from build123d import *

# Parameters (mm, degrees)
EXTRUDE_1_DEPTH     = 20
SKETCH_2_R          = 3.25
CUT_EXTRUDE_1_DEPTH = 115.891252931
SKETCH_3_R          = 3.25
CUT_EXTRUDE_2_DEPTH = 115.891252931
CUT_EXTRUDE_3_DEPTH = 115.891252931
SKETCH_7_R          = 5.5
CUT_EXTRUDE_4_DEPTH = 25
SKETCH_8_R          = 5.5
CUT_EXTRUDE_5_DEPTH = 25


with BuildPart() as part:
    # 草图1 → 凸台-拉伸1 (new body)
    with BuildSketch(Plane(origin=(0, 0, 0), x_dir=(1, 0, 0), z_dir=(0, 1, 0))):
        Polygon((0, 80), (0, 0), (80, 0), (80, 14), (60, 14), (14, 60), (14, 80), align=None)
    extrude(amount=EXTRUDE_1_DEPTH)

    # 草图2 → 切除-拉伸1 (cut, through all)
    with BuildSketch(Plane.ZY):
        with Locations((-70, 10)):
            Circle(SKETCH_2_R)
        with Locations((-50, 10)):
            Circle(SKETCH_2_R)
    extrude(amount=-CUT_EXTRUDE_1_DEPTH, mode=Mode.SUBTRACT)

    # 草图3 → 切除-拉伸2 (cut, through all)
    with BuildSketch(Plane.XY):
        with Locations((70, 10)):
            Circle(SKETCH_3_R)
        with Locations((50, 10)):
            Circle(SKETCH_3_R)
    extrude(amount=-CUT_EXTRUDE_2_DEPTH, mode=Mode.SUBTRACT)

    # 草图4 → 切除-拉伸3 (cut, through all)
    with BuildSketch(Plane.XZ):
        with BuildLine():
            Line((20.901080392, -25.090385961), (31.191934333, -35.381239902))
            Line((31.191934333, -35.381239902), (8.330781791, -58.242392444))
            ThreePointArc((8.330781791, -58.242392444), (6.151201363, -58.675937947), (4.916568228, -56.828178882))
            Line((4.916568228, -56.828178882), (4.916568228, -40.934892559))
            Line((4.916568228, -40.934892559), (20.901080392, -25.090385961))
        make_face()
        with BuildLine():
            Line((24.837924499, -20.930281625), (35.319025282, -31.411382408))
            Line((35.319025282, -31.411382408), (58.210769263, -8.519638426))
            ThreePointArc((58.210769263, -8.519638426), (58.644314766, -6.340057999), (56.796555701, -5.105424864))
            Line((56.796555701, -5.105424864), (40.662781261, -5.105424864))
            Line((40.662781261, -5.105424864), (24.837924499, -20.930281625))
        make_face()
        with BuildLine():
            Line((12.160826912, -5.105424864), (28.651360093, -5.105424864))
            ThreePointArc((28.651360093, -5.105424864), (30.499119158, -6.340057999), (30.065573655, -8.519638426))
            Line((30.065573655, -8.519638426), (8.330781791, -30.254430291))
            ThreePointArc((8.330781791, -30.254430291), (6.151201363, -30.687975793), (4.916568228, -28.840216728))
            Line((4.916568228, -28.840216728), (4.916568228, -12.090508469))
            Line((4.916568228, -12.090508469), (8.000520281, -12.090508469))
            ThreePointArc((8.000520281, -12.090508469), (9.82829842, -15.883616127), (14.030107382, -16.154245149))
            Line((14.030107382, -16.154245149), (12.625484958, -14.430268904))
            ThreePointArc((12.625484958, -14.430268904), (10.638085741, -11.03439689), (14.202657003, -12.700390319))
            Line((14.202657003, -12.700390319), (16.06551283, -13.896467584))
            ThreePointArc((16.06551283, -13.896467584), (15.593703645, -10.049139087), (12.160826912, -8.249167474))
            Line((12.160826912, -8.249167474), (12.160826912, -5.105424864))
        make_face()
    extrude(amount=-CUT_EXTRUDE_3_DEPTH, mode=Mode.SUBTRACT)

    # 草图7 → 切除-拉伸4 (cut)
    with BuildSketch(Plane.XY.offset(-35)):
        with Locations(Location((50, 10, 0), (0, 0, 180))):
            Circle(SKETCH_7_R)
    extrude(amount=CUT_EXTRUDE_4_DEPTH, mode=Mode.SUBTRACT)

    # 草图8 → 切除-拉伸5 (cut)
    with BuildSketch(Plane(origin=(35, 0, 0), x_dir=(0, 0, -1), z_dir=(1, 0, 0))):
        with Locations(Location((50, 10, 0), (0, 0, 180))):
            Circle(SKETCH_8_R)
    extrude(amount=-CUT_EXTRUDE_5_DEPTH, mode=Mode.SUBTRACT)


solid = part.part
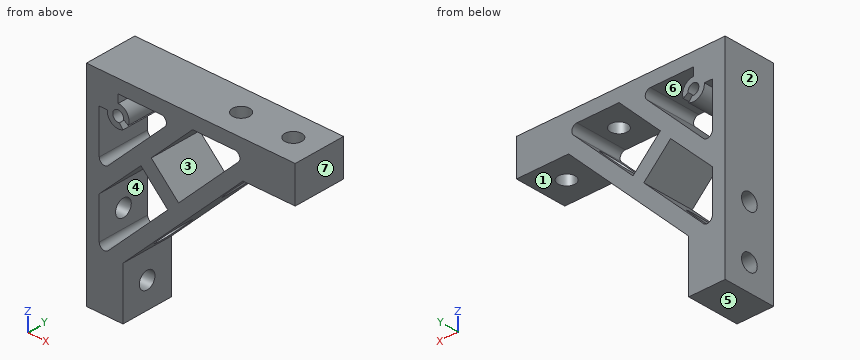
Geometry: final body of the model. Coordinates: model frame, mm. Face numbers are marked on the shaded views. A direction names the side the tool comes from. Give positions to 0.01 mm unless a question says otherwise; leave off trailing zeros. Order: outer loops, then holes, each group sorted by start corner. A loop starts at its lowest first (then second) coordinate and runs counter-clockwise, first axis right, second up. Notation, with made-up numbers: (-36, -0.75) -> (19, -0.75) arc R19 cw to (19, 36.25) -> close; hole circle Ø1 at (-7.75, 63). An arc over 180 degrees is marked (long way). Put each result on its own line as item: value.
Q1. Draft query along Z for the marked faces 4, 5, 6 and 7. Return one class per face: released by +Z, released by -Z, zero draft, split by the parting line, or undercut.
Here are the results:
face 4: undercut
face 5: released by -Z
face 6: undercut
face 7: zero draft
Q2. Pin query (flat end, axial travel): pin 1 (5 mm diameter, centred on x = 50, y = 10, fed in from -Z); pin 2 (7.5 mm diameter, centred on y = 10, z = -50, fed in from +X); pin 3 (6 mm diameter, centred on x = 74.5, y = 13.5, fed in from -Z); pin 4 (8 mm diameter, centred on y = 15, z = -37, fed in from +X). Return the tip coordinate at first contact, or that it passes through.
Here are the results:
pin 1: passes through
pin 2: stops at x = 4.92
pin 3: stops at z = -14
pin 4: stops at x = 41
Q3. Section D-D, the plane z = -50. Return loops of the section in (x, y), then the cut area to 3 significant figures.
Here are the results:
outline: (0, 0) -> (4.92, 0) -> (4.92, 6.75) -> (0, 6.75) -> close; (0, 13.25) -> (4.92, 13.25) -> (4.92, 20) -> (0, 20) -> close; (16.57, 0) -> (24, 0) -> (24, 4.5) -> (16.57, 4.5) -> close; (16.57, 15.5) -> (24, 15.5) -> (24, 20) -> (16.57, 20) -> close
area: 133 mm^2
Q4. Section C-C, the plane y = 17. Count the separate pieces of the cut face and the enclosed holes in it, then the cut area to 3 significant figures.
Here are the results:
separate pieces: 1
enclosed holes: 3
area: 1,910 mm^2
Q5. Section A-A, the plane x = 70. Return loops of the section in (y, z).
Here are the results:
outline: (0, -14) -> (6.75, -14) -> (6.75, 0) -> (0, 0) -> close; (13.25, -14) -> (20, -14) -> (20, 0) -> (13.25, 0) -> close
Q6. Material intervals for L1, parallel to Y at x = 50, z = -23.5; L2, parallel to Y at x = 4.25, z = -70; L3, parallel to X at y = 10, z = -25.25, sorted ascending.
Here are the results:
L1: y = 0 to 4.5, 15.5 to 20
L2: y = 0 to 6.75, 13.25 to 20
L3: x = 0 to 4.92, 13.34 to 20.74, 21.06 to 29.16, 41.48 to 44.5
Q7. Section B-B, the plane z = -70. Return loops of the section in (x, y), then the cut area to 3 significant figures.
Here are the results:
outline: (0, 0) -> (14, 0) -> (14, 6.75) -> (0, 6.75) -> close; (0, 13.25) -> (14, 13.25) -> (14, 20) -> (0, 20) -> close
area: 189 mm^2
Q8. Reachability of the marked faces 1, 2 and 3 from +Z, -Z, +X, -X, +Y, -Y: full face, straight path, thin tool, end or side. Return the list, or none.
Here are the results:
face 1: -Z, +X, +Y, -Y
face 2: +Z, -Z, -X, +Y, -Y
face 3: +Y, -Y
